Geometry: see drawing. Coordinates: mm, zero at the bounding-box minimum. A direction names the side the tool comes from. Give positions to 0.01 mm unless a question says otherwise; leave off trailing zeros. Loops run counter-clockwise (first coordinate to the right, second up) from the corner with the lowest first, then second, coordinate; pieces in that order, holes last. Notation, with made-up numbers: M 24,-29.75 L 70,-29.75 A5 cw 70,-24.75 Z; hole C 29.5,-9.5 d6. An arc over 180 degrees is marked long. Use CSV: the item, a comma, the result in double quotes. Start each with the question number.
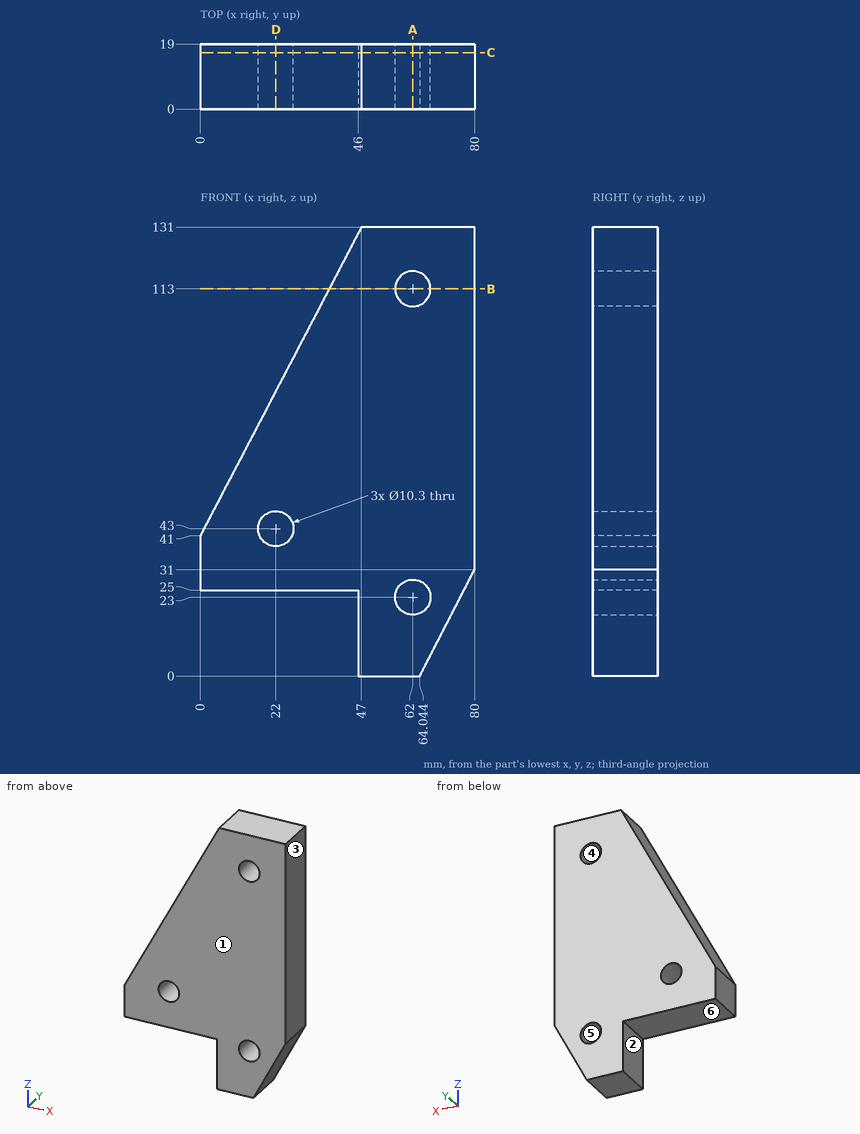
Item 1: Section B-B (z = 113). Output: boundary loops of the cut face in (x, y), then the cut area to 3 significant figures.
Item 2: Section C-C (y = 16.5). Output: boundary loops of the cut face in (x, z).
Item 3: Set-up query: the marked faces 1 and 2. Return all of +Z, -Z, +X, -X, +Y, -Y with unobstructed straight access to the full face (end or side cutting, diameter ignored); none if empty.
Item 4: Material intervals for line 1 (Z direction, x = 62, y = 13); line 2 (X direction, y = 6.25, z = 113); line 3 (Z direction, x = 20, y = 1.25) (1 decimal), sorted ascending.
Item 5: Section A-A (x = 62). Output: boundary loops of the cut face in (y, z), then the cut area to 3 significant figures.
Item 6: First-contact query: pin 1 Ø5.5 at (x, y) = (12.5, 8) entering from -Z; pin 2 Ø4 at (x, z) = (40.5, 75) entering from -Y; pin 3 Ø3 at (y, z) = (5, 72) entering from -X; pin 4 Ø1.5 at (y, z) = (2, 92.5) entering from -X. Flat tips, straight axial feed; report the tip coordinate or a pass-through.
Item 7: Section D-D (x = 22). Output: boundary loops of the cut face in (y, z), then the cut area to 3 significant figures.
Item 8: Mould query, pull axis Z, two halves, no side actions, for the marked faces 3, 4, 5 and 6. Classes: +Z half, -Z half, draft (parallel to the pull), parting line (faces both ways), or undercut.
Recorded:
1,outline,"M 37.6,0 L 56.85,0 L 56.85,19 L 37.6,19 Z; M 67.15,0 L 80,0 L 80,19 L 67.15,19 Z"
1,area,"610 mm²"
2,outline,"M 0,25 L 46,25 L 46,0 L 64.04,0 L 80,31 L 80,131 L 47,131 L 0,41 Z; hole C 22,43 d10.3; hole C 62,23 d10.3; hole C 62,113 d10.3"
3,face 1,"+Z, -Z, +X, -X, -Y"
3,face 2,"-Z, -X, +Y, -Y"
4,line 1,"0 to 17.85, 28.15 to 107.85, 118.15 to 131"
4,line 2,"37.6 to 56.85, 67.15 to 80"
4,line 3,"25 to 38.3, 47.7 to 79.3"
5,outline,"M 0,0 L 19,0 L 19,17.85 L 0,17.85 Z; M 0,28.15 L 19,28.15 L 19,107.85 L 0,107.85 Z; M 0,118.15 L 19,118.15 L 19,131 L 0,131 Z"
5,area,"2,100 mm²"
6,pin 1,"z = 25"
6,pin 2,"y = 0"
6,pin 3,"x = 15.41"
6,pin 4,"x = 26.5"
7,outline,"M 0,25 L 19,25 L 19,37.85 L 0,37.85 Z; M 0,48.15 L 19,48.15 L 19,83.13 L 0,83.13 Z"
7,area,"909 mm²"
8,face 3,"draft"
8,face 4,"undercut"
8,face 5,"undercut"
8,face 6,"-Z half"
